```python
from build123d import *

# Parameters (mm, degrees)
F3_DEPTH       = 3.1
F4_R           = 1
F5_DEPTH       = 9.101
F6_W           = 7
F6_H           = 2.2
F7_DEPTH       = 25
F8_COUNT       = 5
F9_R           = 0.6
F10_DEPTH      = 12.001
F10_DEPTH_BACK = 11.5313382146


with BuildPart() as f1:
    # F0 (on Front) → F1 (revolve)
    with BuildSketch(Plane.XZ):
        Polygon((-3, -7), (-3, 5), (-6, 5), (-6, 0), (-5, 0), (-5, -7), align=None)
    revolve(axis=Axis((0, 0, -4.9457359128), (0, 0, -1)))

    # F2 (on Front) → F3 (join, symmetric)
    with BuildSketch(Plane.XZ):
        with BuildLine():
            ThreePointArc((-7, 2.5), (-7.732233047, 4.267766953), (-9.5, 5))
            ThreePointArc((-9.5, 5), (-12, 2.5), (-9.5, 0))
            ThreePointArc((-9.5, 0), (-7.732233047, 0.732233047), (-7, 2.5))
        make_face()
        with BuildLine():
            Line((-5, 5), (-9.5, 5))
            ThreePointArc((-9.5, 5), (-7.732233047, 4.267766953), (-7, 2.5))
            ThreePointArc((-7, 2.5), (-7.732233047, 0.732233047), (-9.5, 0))
            Line((-9.5, 0), (-5, 0))
            Line((-5, 0), (-5, 5))
        make_face()
    extrude(amount=F3_DEPTH, both=True)

    # F4 (on face) → F5 (cut, through all)
    with BuildSketch(Plane.XZ.offset(3.1)):
        with Locations((-9.5, 2.5)):
            Circle(F4_R)
    extrude(amount=-F5_DEPTH, mode=Mode.SUBTRACT)

    # F6 (on face) → F7 (cut)
    with BuildSketch(Plane.XY.offset(5)):
        with Locations((-9.5, 0)):
            Rectangle(F6_W, F6_H)
    extrude(amount=-F7_DEPTH, mode=Mode.SUBTRACT)

    # F8: F1 ×5 about axis
    f8_axis = Axis((0, 0, -7), (0, 0, 1))


with BuildPart() as f1_1:
    add(f1.part)
    for i in range(1, F8_COUNT):
        add(f1.part.rotate(f8_axis, i * 360 / F8_COUNT))

    # F9 (on Right) → F10 (cut, two sides)
    with BuildSketch(Plane.YZ) as f10_sk:
        with Locations((0, -1.7)):
            Circle(F9_R)
        with Locations((0, -5.3)):
            Circle(F9_R)
    extrude(amount=-F10_DEPTH, mode=Mode.SUBTRACT)
    extrude(f10_sk.sketch, amount=F10_DEPTH_BACK, mode=Mode.SUBTRACT)


solid = f1_1.part
```
Build history of the part. All positions in model axes, mm. A direction names the side the tool comes from. Give positions to 0.01 mm unless a question says otherwise; leave off trailing zeros. Loops run counter-clockwise (first coordinate to the right, second up) from the corner with the lowest first, then second, coordinate; pieces in that order, holes last.
Item 1: Slice it at C-C, the plane z = -1.7. List the corners of the cut face in (x, y), and give its area (3 significant figures).
Answers follow:
outline: (-4.96, -0.6) arc R5 ccw to (4.96, -0.6) - (2.94, -0.6) arc R3 cw to (-2.94, -0.6) - close; (-4.96, 0.6) - (-2.94, 0.6) arc R3 cw to (2.94, 0.6) - (4.96, 0.6) arc R5 ccw to start
area: 45.4 mm2
Item 2: Slice it at D-D, the plane z = 2.5. Give the number of separate pieces and of enclosed holes in the cut face, and give its area (3 significant figures).
Answers follow:
separate pieces: 11
enclosed holes: 1
area: 173 mm2
Item 3: Pull direction Z, two halves, no side cores. Call faces 4 (the face through (-1.84, -5.71, 2.54)), 5 (the face through (0.1, -3.3, -7)), 6 (the face through (-3.955, -0.13, -2.286)): released by +Z, released by -Z, zero draft, split by the parting line, or undercut.
Answers follow:
face 4: zero draft
face 5: released by -Z
face 6: undercut
Item 4: Drill centre lines: line 1 (Y direction, x = 0, z = -1.25); line 2 (X direction, y = -2.75, z = 0.75). Where is each one in solid material? Low to high.
Answers follow:
line 1: y = -5 to -3, 3 to 5
line 2: x = -11.29 to -1.2, 1.2 to 5.42, 5.66 to 9.06
Item 5: Slice it at B-B, the plane y = -1.75. List the corners of the cut face in (x, z), and give its area (3 significant figures).
Answers follow:
outline: (-9.5, 0) - (-4.68, 0) - (-4.68, -7) - (-2.44, -7) - (-2.44, 5) - (-9.5, 5) arc R2.5 ccw to start; (2.44, -7) - (4.68, -7) - (4.68, 0) - (7.68, 0) - (7.68, 5) - (2.44, 5) - close; hole circle Ø2 at (-9.5, 2.5)
area: 99.7 mm2
Item 6: Which spindle directions (+Z, -Z, +X, -X, +Y, -Y) get a long thin tool onto all of the face, cutting with end or side? Do faces 1 (the face through (-8, -3.1, 3)), 2 (the face through (0.52, 8.43, 2.54)), 3 (the face through (6.129, -5.813, 3.091)). Say none if no direction does.
Answers follow:
face 1: +Z, -Z, -X
face 2: +Z, -Z, +Y
face 3: +Z, -Z
Item 7: Flat gauge pins, fed straight in: pin 1 (1.9 mm diameter, centred on y = 0, z = -5.3, fed in from -X); pin 2 (2.5 mm diameter, centred on x = -9.5, z = 2.5, fed in from -Y); pin 3 (1.6 mm diameter, centred on y = 0, z = -1.7, fed in from +X). Where does each tip first touch, or does it go through?
Answers follow:
pin 1: stops at x = -5
pin 2: stops at y = -3.1
pin 3: stops at x = 5
Item 8: Slice it at A-A, the plane x = -7.75. List the corners of the cut face in (y, z), and give its area (3 significant figures).
Answers follow:
outline: (-3.1, 0) - (-1.1, 0) - (-1.1, 5) - (-3.1, 5) - close; (1.1, 0) - (3.1, 0) - (3.1, 5) - (1.1, 5) - close
area: 20.0 mm2
